The listing builds one solid part. Answer for the finished solid, in the listing's coordinates (mm). A direction names the side the tool comes from. Give positions to 0.01 mm unless a question says otherwise; leave off trailing zeros. Write each loop counter-clockwise with the first axis right and the second up, starting at its lowest first coordinate (ties: lowest second). Pieces come first, ordered by that corner, then holes. Notation, with made-up numbers: (25, 75) - (82, 75) arc R10 cw to (82, 83) - close; hole circle Ø10 at (-28, -34.75). An arc over 180 degrees is marked (long way). Write each question's results on one line, items separated by ' | '. Start each with the question number.
Q1. Section A-A (y = 0) is taken. Determine the outline of the cut face in (x, z).
Q2. For a pull along X with two mould halves and no side action, classify faces 4 (the face through (-6.75, 0, 0)), 5 (the face through (-3, 0, 1)), 6 (the face through (6.75, 0, 0)), 7 (the face through (-2, 0, -14.8)) as pulls with the +X half, pulls with the -X half, needs draft (parallel to the pull), parting line crosses it, or undercut.
Q3. Section C-C (x = 2.25) is taken. Determine the outline of the cut face in (y, z), plus the area to 3 significant figures.
Q4. For faces 1 (the face through (1.3, -1.3, -14)), 2 (the face through (-1.5, 0.07, -14.39)), 3 (the face through (0.99, 6.13, -6.94)), determine the directions among +Z, -Z, +X, -X, +Y, -Y from which every point of the face is accessible in a straight line to the end or side of a thin tool.
Q5. Section B-B (z = -3.25) is taken. Determine the outline of the cut face in (x, y).
Q6. Flat-ended cylindrical pins translate along their axes: pin 1 Ø3 at (x, y) = (0, 1) entering from +Z; pin 2 Ø1.5 at (x, z) = (0, 7.3) entering from +Y; pin 3 Ø1.8 at (x, y) = (0, 0) entering from -Z. Find the tip coordinate at first contact, or state that the pin passes through.
Q7. Find the intervals of material crossed by probe 1 along X at (y, z) = (6.3, 7.3); probe 2 along Z at (x, y) = (0, 6.4); probe 3 along Z at (x, y) = (-1.5, -1.25), in increasing order.
```python
from build123d import *

# Parameters (mm, degrees)
SKETCH1_W                 = 13.5
SKETCH1_H                 = 15
BOSS_EXTRUDE1_DEPTH       = 14.8
SKETCH2_R                 = 3
CUT_EXTRUDE1_DEPTH        = 28.8
SKETCH3_R                 = 1.5
CUT_EXTRUDE2_DEPTH        = 30.6
M3X0_5_TAPPED_HOLE1_D     = 2.5
M3X0_5_TAPPED_HOLE1_DEPTH = 2.7
M3X0_5_TAPPED_HOLE1_TIP   = 0.751075774


with BuildPart() as part:
    # Sketch1 → Boss-Extrude1 (new body, symmetric)
    with BuildSketch(Plane.XY):
        Rectangle(SKETCH1_W, SKETCH1_H)
    extrude(amount=BOSS_EXTRUDE1_DEPTH, both=True)

    # Sketch2 → Cut-Extrude1 (cut)
    with BuildSketch(Plane.XY.offset(14.8)):
        Circle(SKETCH2_R)
    extrude(amount=-CUT_EXTRUDE1_DEPTH, mode=Mode.SUBTRACT)

    # Sketch3 → Cut-Extrude2 (cut, through all)
    with BuildSketch(Plane.XY.offset(14.8)):
        Circle(SKETCH3_R)
    extrude(amount=-CUT_EXTRUDE2_DEPTH, mode=Mode.SUBTRACT)

    # M3x0.5 Tapped Hole1
    with Locations(Plane(origin=(0, 7.5, 0), x_dir=(1, 0, 0), z_dir=(0, 1, 0))):
        with Locations((0, 7.7), (0, -7.3)):
            Hole(M3X0_5_TAPPED_HOLE1_D / 2, depth=M3X0_5_TAPPED_HOLE1_DEPTH)
            with Locations((0, 0, -(M3X0_5_TAPPED_HOLE1_DEPTH + M3X0_5_TAPPED_HOLE1_TIP / 2))):  # 118° drill point
                Cone(0, M3X0_5_TAPPED_HOLE1_D / 2, M3X0_5_TAPPED_HOLE1_TIP, mode=Mode.SUBTRACT)


solid = part.part
```
Answers below:
1) outline: (-6.75, -14.8) - (-1.5, -14.8) - (-1.5, -14) - (-3, -14) - (-3, 14.8) - (-6.75, 14.8) - close; (1.5, -14.8) - (6.75, -14.8) - (6.75, 14.8) - (3, 14.8) - (3, -14) - (1.5, -14) - close
2) face 4: pulls with the -X half | face 5: undercut | face 6: pulls with the +X half | face 7: needs draft
3) outline: (-7.5, -14.8) - (7.5, -14.8) - (7.5, 14.8) - (1.98, 14.8) - (1.98, -14) - (-1.98, -14) - (-1.98, 14.8) - (-7.5, 14.8) - close | area: 330 mm2
4) face 1: +Z | face 2: +Z, -Z | face 3: +Y
5) outline: (-6.75, -7.5) - (6.75, -7.5) - (6.75, 7.5) - (-6.75, 7.5) - close; hole circle Ø6 at (0, 0)
6) pin 1: stops at z = -14 | pin 2: stops at y = 4.5 | pin 3: passes through
7) probe 1: x = -6.75 to -1.25, 1.25 to 6.75 | probe 2: z = -14.8 to -8.95, -6.45 to 6.05, 8.55 to 14.8 | probe 3: z = -14.8 to -14
